```python
from build123d import *

# Parameters (mm, degrees)
SKETCH1_W                = 12.69619
SKETCH1_H                = 3.175
SKETCH2_R                = 6.34619
BOSS_EXTRUDE1_DEPTH      = 2.032
M2_5_CLEARANCE_HOLE1_D   = 2.7051
M3_CLEARANCE_HOLE1_D     = 3.556
M3_CLEARANCE_HOLE1_DEPTH = 5.207
SKETCH9_R                = 3.175
CUT_EXTRUDE1_DEPTH       = 19.694901177


with BuildPart() as part:
    # Sketch1 → Revolve1 (revolve)
    with BuildSketch(Plane.XY, mode=Mode.PRIVATE) as revolve1_sk:
        with Locations((6.348095, 1.5875)):
            Rectangle(SKETCH1_W, SKETCH1_H)
    revolve(revolve1_sk.sketch.rotate(Axis((0, 3.175, 0), (0, -1, 0)), 270), axis=Axis((0, 3.175, 0), (0, -1, 0)))

    # Sketch2 → Boss-Extrude1 (add)
    with BuildSketch(Plane(origin=(0, 3.175, 0), x_dir=(-1, 0, 0), z_dir=(0, 1, 0))):
        with Locations(Location((0, 0, 0), (0, 0, 90))):
            Circle(SKETCH2_R)
    extrude(amount=BOSS_EXTRUDE1_DEPTH)

    # M2.5 Clearance Hole1 (through all)
    with Locations(Plane(origin=(0, 3.175, 0), x_dir=(1, 0, 0), z_dir=(0, 1, 0))):
        with Locations((-9.779, 0), (0, 9.779), (9.779, 0), (0, -9.779)):
            Hole(M2_5_CLEARANCE_HOLE1_D / 2)

    # M3 Clearance Hole1
    with Locations(Plane(origin=(0, 0, 0), x_dir=(-1, 0, 0), z_dir=(0, -1, 0))):
        with Locations((6.914797213, 6.914797213), (-6.914797213, 6.914797213), (-6.914797213, -6.914797213), (6.914797213, -6.914797213)):
            Hole(M3_CLEARANCE_HOLE1_D / 2, depth=M3_CLEARANCE_HOLE1_DEPTH)

    # Sketch9 → Cut-Extrude1 (cut, through all)
    with BuildSketch(Plane(origin=(0, 5.207, 0), x_dir=(1, 0, 0), z_dir=(0, 1, 0))):
        with Locations(Location((0, 0, 0), (0, 0, 270))):
            Circle(SKETCH9_R)
    extrude(amount=-CUT_EXTRUDE1_DEPTH, mode=Mode.SUBTRACT)


solid = part.part
```
Could you check a few things on this model? Use its own coordinates, in mm. A direction names the side the tool comes from. Round coordinates to 2 decimals unless told otherwise and drop trailing zeros. Write each loop counter-clockwise with the first axis right and the second up, starting at its lowest first coordinate (ties: lowest second). Pieces come first, ordered by that corner, then holes. Notation, with made-up numbers: M -29.5,1.5 L -14.5,1.5 A20 ccw -14.5,35.5 Z; hole C 87,42.5 d2. An arc over 180 degrees is marked long. Write each question's results on one line, items separated by ' | '. Start each with the question number.
1. Imagine slicing it at A-A on x = 0. List the corners of the cut face in (y, z) for me (3 decimals), and give its area (3 significant figures).
2. I'm going to push flat-ended pins straight in: pin 1 Ø2 at (x, y) = (-6, 1.5) entering from +Z; pin 2 Ø2 at (x, y) = (7.5, 3) entering from +Z; pin 3 Ø3 at (x, z) = (6.91, -6.91) entering from +Y; pin 4 Ø2 at (y, z) = (4.5, 0.5) entering from -X. Where does each tip first touch, or does it pass through?
3. Imagine slicing it at C-C on x = 10.5. List the corners of the cut face in (y, z) for me (3 decimals), and give its area (3 significant figures).
4. On a 3-axis mill with a long thin cutter (end or side, diameter ignored), from which of +Z, -Z, +X, -X, +Y, -Y can I reach the whole of each face in a straight line? I mean faces 1 (the face through (-3, 3.175, -6)), 2 (the face through (-1.93, 2.64, -2.52)). Say none if no direction works.
5. Imagine slicing it at B-B on z = 0. List the corners of the cut face in (x, y) for me (3 decimals).
6. Thinking about a two-plate mould opening in X: for faces 3 (the face through (6.29, 4.18, -0.83)), 4 (the face through (-3, 0, 3)), 5 (the face through (0.29, 1.57, 11.1)), which applies, +X half, -X half, draft (parallel to the pull), parting line (faces both ways), or undercut?
7. Imagine slicing it at D-D on y = 1.6. Count the separate pieces of the cut face and the enclosed holes in it, and give its area (3 significant figures).
8. I need wall thicknesses on L1, parallel to Z at x = -6, y = 0.4; L2, parallel to Y at x = 5.5, z = 4.5 (3 decimals); L3, parallel to Z at x = -7, y = 1.95. Which ranges of each line are inside material? Lowest first, please. Write a range as from..to.
Result sheet:
1) outline: M 0,-12.696 L 3.175,-12.696 L 3.175,-11.132 L 0,-11.132 Z; M 0,-8.426 L 3.175,-8.426 L 3.175,-6.346 L 5.207,-6.346 L 5.207,-3.175 L 0,-3.175 Z; M 0,3.175 L 5.207,3.175 L 5.207,6.346 L 3.175,6.346 L 3.175,8.426 L 0,8.426 Z; M 0,11.132 L 3.175,11.132 L 3.175,12.696 L 0,12.696 Z | area: 56.2 mm^2
2) pin 1: stops at z = 11.67 | pin 2: stops at z = 10.91 | pin 3: passes through | pin 4: stops at x = -6.35
3) outline: M 0,-7.137 L 3.175,-7.137 L 3.175,-1.144 L 0,-1.144 Z; M 0,1.144 L 3.175,1.144 L 3.175,7.137 L 0,7.137 Z | area: 38.1 mm^2
4) face 1: +Y | face 2: +Y, -Y
5) outline: M -12.696,0 L -11.132,0 L -11.132,3.175 L -12.696,3.175 Z; M -8.426,0 L -3.175,0 L -3.175,5.207 L -6.346,5.207 L -6.346,3.175 L -8.426,3.175 Z; M 3.175,0 L 8.426,0 L 8.426,3.175 L 6.346,3.175 L 6.346,5.207 L 3.175,5.207 Z; M 11.132,0 L 12.696,0 L 12.696,3.175 L 11.132,3.175 Z
6) face 3: parting line | face 4: draft | face 5: undercut
7) separate pieces: 1 | enclosed holes: 9 | area: 412 mm^2
8) L1: z = -11.19..-8.44, -5.39..5.39, 8.44..11.19 | L2: y = 0..3.175 | L3: z = -10.59..-8.69, -5.14..5.14, 8.69..10.59
